Read the model definition and answer for the solid it produces. Units are mm, in the model's axes. Face numbers are marked on the shaded views. A direction names the side the tool comes from. Coordinates: 2 decimals unless noted, no trailing zeros. Order: outer loops, then holes, each group sorted by start corner. A loop starts at its lowest first (then second) coordinate and runs counter-clockwise, first axis right, second up. Notation, with made-up numbers: (36.25, 42.5) -> (90.25, 42.5) arc R14 cw to (90.25, 58.5) -> close; hole circle Ø6 at (-9, 42.5). An arc over 180 degrees is marked (long way). Answer as a JSON object with one key per item and string values. Group by question number.
1) Determine the mould class of the marked faces 1, 2, 3 and 4 for opening direction Y: released by +Y, released by -Y, zero draft, split by the parting line, or undercut.
2) Section C-C on x = -358.5 is taken. Determine the outline of the cut face in (y, z), and give its area (3 significant figures).
3) A tool of negligible diameter and unlimited length cuts with its end or side. For the marked faces 5, 6, 7, 8 and 9, from which of +Z, -Z, +X, -X, +Y, -Y can it reach the whole face along a straight path? Write none if from no direction.
4) Given pin 1 (6 mm diameter, centred on y = -473, z = 115.5, fed in from +X), flat-ended and moving along its own axis, determine where the tip first touches the part or whether it passes through.
5) Section D-D on z = 150 is taken. Determine the outline of the cut face in (x, y).
6) Section A-A on y = -38.5 is taken. Determine the outline of the cut face in (x, z).
7) Consider L1, parallel to X at y = -306.5, z = -260; L2, parallel to X at y = -514, z = -225; L3, parallel to Y at x = -343, z = 150. Determine where each line is inside the solid, lowest interval first.
8) Section B-B on y = -345.5 is taken. Determine the outline of the cut face in (x, z).
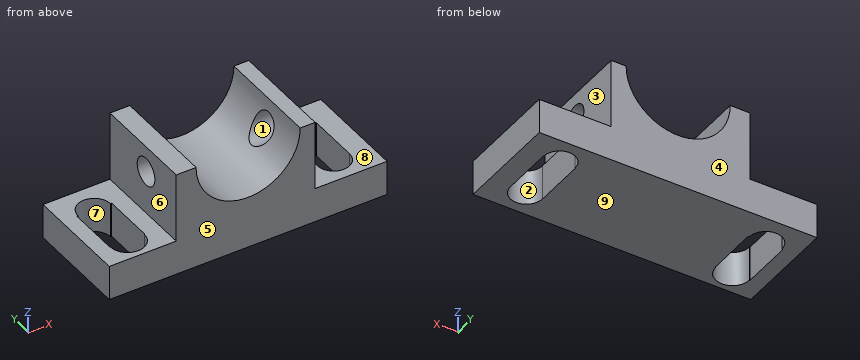
from build123d import *

# Parameters (mm, degrees)
F1_DEPTH = 600
F2_R     = 80
F3_DEPTH = 1185.644113
F6_DEPTH = 200.001


with BuildPart() as f1:
    # F0 (on Front) → F1 (new body)
    with BuildSketch(Plane.XZ):
        with BuildLine():
            Line((-800, -300), (800, -300))
            Line((800, -300), (800, -100))
            Line((800, -100), (385.643113, -100))
            Line((385.643113, -100), (385.643113, 300))
            Line((385.643113, 300), (300, 300))
            ThreePointArc((300, 300), (0, 0), (-300, 300))
            Line((-300, 300), (-414.356887, 300))
            Line((-414.356887, 300), (-414.356887, -100))
            Line((-414.356887, -100), (-800, -100))
            Line((-800, -100), (-800, -300))
        make_face()
    extrude(amount=F1_DEPTH)

    # F2 (on face) → F3 (cut, through all)
    with BuildSketch(Plane.YZ.offset(385.643113)):
        with Locations((-326.723337, 150)):
            Circle(F2_R)
    extrude(amount=-F3_DEPTH, mode=Mode.SUBTRACT)

    # F5 (on face) → F6 (cut, through all)
    with BuildSketch(Plane.XY.offset(-100)):
        with BuildLine():
            Line((679.844578, -450.278306), (679.844578, -150.278306))
            Line((679.844578, -150.278306), (677.441342, -150.278306))
            ThreePointArc((677.441342, -150.278306), (587.536824, -60.373787), (497.632305, -150.278306))
            Line((497.632305, -150.278306), (495.22907, -150.278306))
            Line((495.22907, -150.278306), (495.22907, -450.278306))
            ThreePointArc((495.22907, -450.278306), (587.536824, -542.58606), (679.844578, -450.278306))
        make_face()
        with BuildLine():
            Line((-512.387931, -469.733909), (-512.387931, -169.733909))
            Line((-512.387931, -169.733909), (-519.35312, -169.733909))
            ThreePointArc((-519.35312, -169.733909), (-612.463176, -76.623852), (-705.573233, -169.733909))
            Line((-705.573233, -169.733909), (-712.538421, -169.733909))
            Line((-712.538421, -169.733909), (-712.538421, -469.733909))
            Line((-712.538421, -469.733909), (-709.608744, -469.733909))
            ThreePointArc((-709.608744, -469.733909), (-612.463176, -566.879477), (-515.317608, -469.733909))
            Line((-515.317608, -469.733909), (-512.387931, -469.733909))
        make_face()
    extrude(amount=-F6_DEPTH, mode=Mode.SUBTRACT)


solid = f1.part
Worked answers:
{
 "1": {"face 1": "undercut", "face 2": "undercut", "face 3": "zero draft", "face 4": "released by +Y"},
 "2": {"outline": "(-600, -300) -> (0, -300) -> (0, 300) -> (-600, 300) -> close; hole circle Ø160 at (-326.72, 150)", "area": "340,000 mm²"},
 "3": {"face 5": "+Z, -Z, +X, -X, -Y", "face 6": "+Z, -X, +Y, -Y", "face 7": "+Z, -Z", "face 8": "+Z, +X, +Y, -Y", "face 9": "-Z, +X, -X, +Y, -Y"},
 "4": {"pin 1": "stops at x = 385.64"},
 "5": {"outline": "(-414.36, -600) -> (-259.81, -600) -> (-259.81, -406.72) -> (-414.36, -406.72) -> close; (-414.36, -246.72) -> (-259.81, -246.72) -> (-259.81, 0) -> (-414.36, 0) -> close; (259.81, -600) -> (385.64, -600) -> (385.64, -406.72) -> (259.81, -406.72) -> close; (259.81, -246.72) -> (385.64, -246.72) -> (385.64, 0) -> (259.81, 0) -> close"},
 "6": {"outline": "(-800, -300) -> (800, -300) -> (800, -100) -> (385.64, -100) -> (385.64, 300) -> (300, 300) arc R300 cw to (-300, 300) -> (-414.36, 300) -> (-414.36, -100) -> (-800, -100) -> close"},
 "7": {"L1": "x = -800 to -712.54, -512.39 to 495.23, 679.84 to 800", "L2": "x = -800 to -698.94, -525.99 to 520.75, 654.32 to 800", "L3": "y = -600 to -406.72, -246.72 to 0"},
 "8": {"outline": "(-800, -300) -> (-712.54, -300) -> (-712.54, -100) -> (-800, -100) -> close; (-512.39, -300) -> (495.23, -300) -> (495.23, -100) -> (385.64, -100) -> (385.64, 72.23) -> (195.25, 72.23) arc R300 cw to (-195.25, 72.23) -> (-414.36, 72.23) -> (-414.36, -100) -> (-512.39, -100) -> close; (-414.36, 227.77) -> (-291.17, 227.77) arc R300 cw to (-300, 300) -> (-414.36, 300) -> close; (291.17, 227.77) -> (385.64, 227.77) -> (385.64, 300) -> (300, 300) arc R300 cw to start; (679.84, -300) -> (800, -300) -> (800, -100) -> (679.84, -100) -> close"}
}
